from build123d import *

# Parameters (mm, degrees)
SKETCH1_W                      = 16
SKETCH1_H                      = 16
BOSS_EXTRUDE1_DEPTH            = 8
BOSS_EXTRUDE2_START            = -3.3
BOSS_EXTRUDE2_DEPTH            = 4.7
CBORE_FOR_M3_SHCS1_D           = 4
CBORE_FOR_M3_SHCS1_CBORE_D     = 5.5
CBORE_FOR_M3_SHCS1_CBORE_DEPTH = 2.5
WIRECLEARANCE_SIZE             = 2.5
EDGEBREAK_0_1_SIZE             = 0.1


with BuildPart() as part:
    # Sketch1 → Boss-Extrude1 (new body)
    with BuildSketch(Plane(origin=(0, 0, 0), x_dir=(1, 0, 0), z_dir=(0, 1, 0))):
        Rectangle(SKETCH1_W, SKETCH1_H)
        with BuildLine():
            Line((-4.624026974, -1.974939831), (-2.324025974, -4.374940831))
            Line((-2.324025974, -4.374940831), (2.375974026, -4.374940831))
            Line((2.375974026, -4.374940831), (4.575973243, -1.974939653))
            ThreePointArc((4.575973243, -1.974939653), (2.765999996, 0.025060065), (4.575975026, 2.025058169))
            Line((4.575975026, 2.025058169), (2.375974026, 4.425059169))
            Line((2.375974026, 4.425059169), (-2.324025974, 4.425059169))
            Line((-2.324025974, 4.425059169), (-4.624764746, 2.025131808))
            ThreePointArc((-4.624764746, 2.025131808), (-2.814051979, 0.025429887), (-4.624026974, -1.974939831))
        make_face(mode=Mode.SUBTRACT)
    extrude(amount=-BOSS_EXTRUDE1_DEPTH)

    # Sketch2 → Boss-Extrude2 (add)
    with BuildSketch(Plane(origin=(0, 0, 0), x_dir=(1, 0, 0), z_dir=(0, 1, 0)).offset(BOSS_EXTRUDE2_START)):
        with BuildLine():
            ThreePointArc((3.992847908, -2.611076921), (6.420495716, -2.179038926), (7.525974026, 0.025059169))
            ThreePointArc((7.525974026, 0.025059169), (6.420496186, 2.229156913), (3.992849032, 2.661195592))
            Line((3.992849032, 2.661195592), (4.575975026, 2.025058169))
            ThreePointArc((4.575975026, 2.025058169), (2.765999996, 0.025060065), (4.575973243, -1.974939653))
            Line((4.575973243, -1.974939653), (3.992847908, -2.611076921))
        make_face()
        with BuildLine():
            Line((4.575975026, 2.025058169), (3.992849032, 2.661195592))
            ThreePointArc((3.992849032, 2.661195592), (2.025974026, 0.025059755), (3.992847908, -2.611076921))
            Line((3.992847908, -2.611076921), (4.575973243, -1.974939653))
            ThreePointArc((4.575973243, -1.974939653), (2.765999996, 0.025060065), (4.575975026, 2.025058169))
        make_face()
        with BuildLine():
            ThreePointArc((-4.020334349, -2.604879951), (-2.613522415, -1.610842422), (-2.074025974, 0.025059169))
            ThreePointArc((-2.074025974, 0.025059169), (-2.61366584, 1.661154545), (-4.020795486, 2.655139164))
            Line((-4.020795486, 2.655139164), (-4.624764746, 2.025131808))
            ThreePointArc((-4.624764746, 2.025131808), (-2.814051979, 0.025429887), (-4.624026974, -1.974939831))
            Line((-4.624026974, -1.974939831), (-4.020334349, -2.604879951))
        make_face()
        with BuildLine():
            Line((-4.624764746, 2.025131808), (-4.020795486, 2.655139164))
            ThreePointArc((-4.020795486, 2.655139164), (-7.574025963, 0.024818081), (-4.020334349, -2.604879951))
            Line((-4.020334349, -2.604879951), (-4.624026974, -1.974939831))
            ThreePointArc((-4.624026974, -1.974939831), (-2.814051979, 0.025429887), (-4.624764746, 2.025131808))
        make_face()
    extrude(amount=-BOSS_EXTRUDE2_DEPTH)

    # CBORE for M3 SHCS1 (through all)
    with Locations(Plane(origin=(0, 0, 0), x_dir=(1, 0, 0), z_dir=(0, 1, 0))):
        with Locations((4.775974026, 0.025059169), (-4.824025974, 0.025059169)):
            CounterBoreHole(CBORE_FOR_M3_SHCS1_D / 2, CBORE_FOR_M3_SHCS1_CBORE_D / 2, CBORE_FOR_M3_SHCS1_CBORE_DEPTH)

    # WireClearance
    wireclearance_edges = [part.edges().sort_by_distance(p)[0] for p in [
        (0.025974026, -8, -4.425059169),
        (0.025974026, -8, 4.374940831),
    ]]
    chamfer(wireclearance_edges, length=WIRECLEARANCE_SIZE)

    # Edgebreak-0.1
    edgebreak_0_1_edges = [part.edges().sort_by_distance(p)[0] for p in [
        (-8, -8, 0),
        (0.025974026, -5.5, -4.425059169),
        (0.025974026, -5.5, 4.374940831),
        (0, -8, 8),
        (-1.974073017, -8, -4.790099166),
        (2.038578604, -8, 4.743008876),
        (0.025974026, 0, 4.374940831),
        (3.184410967, 0, 3.493008876),
        (0.025974026, 0, -4.425059169),
        (-3.17241073, 0, -3.540099167),
        (8, -8, 0),
        (2.038578152, -8, -4.793127381),
        (0, 0, 8),
        (-8, 0, 0),
        (0, 0, -8),
        (-1.974263473, -8, 4.739910391),
        (8, 0, 0),
        (0, -8, -8),
        (-3.172180161, 0, 3.489910391),
        (-7.574025963, 0, -0.024818081),
        (8, -4, 8),
        (-8, -4, 8),
        (-8, -4, -8),
        (8, -4, -8),
        (-2.824025974, -8, -0.025059169),
        (3.184411529, 0, -3.543127381),
        (7.525974026, 0, -0.025058583),
        (6.775974026, -8, -0.025059169),
    ]]
    chamfer(edgebreak_0_1_edges, length=EDGEBREAK_0_1_SIZE)


solid = part.part
The listing builds one solid part. Answer for the finished solid, in the listing's coordinates (mm). A direction names the side the tool comes from. Give positions to 0.01 mm unless a question says otherwise; leave off trailing zeros. Write each loop counter-clockwise with the first axis right and the second up, starting at its lowest first coordinate (ties: lowest second). Pieces come first, ordered by that corner, then holes.
Item 1: Section D-D, the plane z = -1 is taken. Count the separate pieces of the cut face and the enclosed holes in it, plus the area to 3 significant figures.
Item 2: A flat-ended cylindrical pin translates along its axis: P1, Ø2.5, axis at x = -6, z = 0, coming from the +Y side. Find the tip coordinate at first contact, or state that the pin passes through.
Item 3: Which of the six approach directions +Z, -Z, +X, -X, +Y, -Y give full straight-line access (tool end or side, diameter ignored) to faces 1 (the flat face through (0, -4, -8)), 2 (the flat face through (-0.005, -6.498, 5.373)), 3 (the flat face through (7, -2.5, 1))?
Item 4: Section A-A, the plane x = -1.75 is taken. Write down the section's boundary in (y, z), plus the area to 3 significant figures.
Item 5: Find the intervals of material crossed by line 1 along Z through (x, y) = (-4.75, -0.5); line 2 along Z through (x, y) = (1, -1.5); line 3 along X through (y, z) = (-3.75, -0.75), in increasing order.
Item 6: Section C-C, the plane y = -2.25 is taken. Write down the section's boundary in (x, z).
Item 7: Determine the mould class of faces 4 (the flat face through (-8, -4, 0)), 5 (the flat face through (0, -4, 8)), 6 (the flat face through (2.896, -3.945, -3.858)) for opening direction X: released by +X, released by -X, zero draft, split by the parting line, or undercut.
Item 8: Section B-B, the plane y = -4.5 is taken. Write down the section's boundary in (x, z), plus the area to 3 significant figures.
Completed:
1. separate pieces: 4
1. enclosed holes: 0
1. area: 26.9 mm2
2. P1: stops at y = -2.5
3. face 1: -Z, +X, -X, +Y, -Y
3. face 2: -Y
3. face 3: +Y
4. outline: (-8, -7.9) - (-7.9, -8) - (-0.1, -8) - (0, -7.9) - (0, -4.53) - (-0.1, -4.43) - (-5.4, -4.43) - (-5.57, -4.5) - (-6.1, -5.02) - (-7.9, -5.02) - (-8, -5.17) - close; (-8, 5.12) - (-7.9, 4.97) - (-6.1, 4.97) - (-5.57, 4.45) - (-5.4, 4.37) - (-0.1, 4.37) - (0, 4.47) - (0, 7.9) - (-0.1, 8) - (-7.9, 8) - (-8, 7.9) - close
4. area: 54.9 mm2
5. line 1: z = -8 to -2.77, 2.72 to 8
5. line 2: z = -8 to -4.43, 4.37 to 8
5. line 3: x = -8 to -6.69, -2.96 to -2.17, 2.12 to 2.91, 6.64 to 8
6. outline: (-8, -7.9) - (-7.9, -8) - (7.9, -8) - (8, -7.9) - (8, 7.9) - (7.9, 8) - (-7.9, 8) - (-8, 7.9) - close; hole (-4.02, -2.66) - (-2.32, -4.43) - (2.38, -4.43) - (3.99, -2.66) arc R2.75 ccw (long way) to (3.99, 2.61) - (2.38, 4.37) - (-2.32, 4.37) - (-4.02, 2.6) arc R2.75 ccw (long way) to start
7. face 4: released by -X
7. face 5: zero draft
7. face 6: undercut
8. outline: (-8, -7.9) - (-7.9, -8) - (7.9, -8) - (8, -7.9) - (8, 7.9) - (7.9, 8) - (-7.9, 8) - (-8, 7.9) - close; hole circle Ø4 at (-4.82, -0.03); hole (-4.02, -2.66) - (-2.32, -4.43) - (2.38, -4.43) - (3.99, -2.66) arc R2.75 cw to (3.99, 2.61) - (2.38, 4.37) - (-2.32, 4.37) - (-4.02, 2.6) arc R2.75 cw to start; hole circle Ø4 at (4.78, -0.03)
8. area: 181 mm2
